```python
from build123d import *

# Parameters (mm, degrees)
FILLET1_R          = 0.75
CUT_EXTRUDE6_DEPTH = 3


with BuildPart() as part:
    # Sketch1 → Revolve1 (revolve)
    with BuildSketch(Plane(origin=(0, 0, 0), x_dir=(0, 0, -1), z_dir=(1, 0, 0))):
        with BuildLine():
            Line((0, 0), (140, 0))
            Line((140, 0), (140, 4.75))
            Line((140, 4.75), (6.25, 4.75))
            Line((6.25, 4.75), (6.25, 8.15))
            ThreePointArc((6.25, 8.15), (1.742375921, 5.135294539), (0, 0))
        make_face()
    revolve(axis=Axis((0, 0, 0), (0, 0, -1)))

    # Fillet1
    fillet1_edges = [part.edges().sort_by_distance(p)[0] for p in [
        (0, -8.15, -6.25),
        (0, -4.75, -140),
    ]]
    fillet(fillet1_edges, radius=FILLET1_R)

    # Sketch4 → Cut-Extrude6 (cut)
    with BuildSketch(Plane.XY):
        with BuildLine():
            Line((1.875, -3.247595264), (1.875, -9.329244328))
            Line((1.875, -9.329244328), (-1.875, -9.329244328))
            Line((-1.875, -9.329244328), (-1.875, -3.247595264))
            ThreePointArc((-1.875, -3.247595264), (-3.75, 0), (-1.875, 3.247595264))
            Line((-1.875, 3.247595264), (-1.875, 9.329244328))
            Line((-1.875, 9.329244328), (1.875, 9.329244328))
            Line((1.875, 9.329244328), (1.875, 3.247595264))
            ThreePointArc((1.875, 3.247595264), (3.75, 0), (1.875, -3.247595264))
        make_face()
    extrude(amount=-CUT_EXTRUDE6_DEPTH, mode=Mode.SUBTRACT)


solid = part.part
```
Can you work these out from the model? Positions are in its coordinate system, mm. A direction names the side the tool comes from. Round coordinates to 2 decimals unless told otherwise and drop trailing zeros. Loops run counter-clockwise (first coordinate to the right, second up) from the corner with the lowest first, then second, coordinate; pieces in that order, holes last. Notation, with made-up numbers: (65.25, 40.5) -> (87.25, 40.5) arc R21 ccw to (87.25, 68.5) -> close; hole circle Ø7 at (-21.5, -22). An arc over 180 degrees is marked (long way). One line per item, written item: value. Start each with the question number.
1. For faces 1 (the cylindrical face through (3.75, 0.05, -1.92)), 2 (the flat face through (-5, 1, -6.25)), 3 (the flat face through (-1.875, 4, -2)), which set-ups out of +Z, -Z, +X, -X, +Y, -Y let a thin tool reach every point of the face, with its end or its side?
2. If we section it at A-A, the plane z = -98: Write out the boundary of the cut face in (x, y).
3. For pin 1 (6 mm diameter, centred on y = -3.5, z = -96, fed in from +X); pin 2 (1.5 mm diameter, centred on x = 0, z = -85.5, fed in from -Y); pin 3 (2.5 mm diameter, centred on y = 5.5, z = -2.5, fed in from -X), each with a flat end and sliding along its axis, tell me the tip position at first contact or that it passes through.
4. If I drill on probe 1 along Y at (x, z) = (0.25, -9.5); probe 2 along Z at (x, y) = (3.25, -1.25); probe 3 along X at (y, z) = (-0.5, -103), over which ranges is the centre line in solid material (lowest first)?
5. If we mould it in two halves opening along X, with no side actions, what happens to faces 4 (the flat face through (0, 0, -140)), 5 (the cylindrical face through (-4.214, 2.192, -71.819)), 6 (the cylindrical face through (-3.75, -0.05, -1.92))? For each: pulls with the +X half, pulls with the -X half, needs draft (parallel to the pull), parting line crosses it, or undercut.
Calculated:
1. face 1: +Z
1. face 2: -Z
1. face 3: +Z, +Y, -Y
2. outline: circle Ø9.5 at (0, 0)
3. pin 1: stops at x = 4.72
3. pin 2: stops at y = -4.75
3. pin 3: stops at x = -4.94
4. probe 1: y = -4.74 to 4.74
4. probe 2: z = -140 to -3
4. probe 3: x = -4.72 to 4.72
5. face 4: needs draft
5. face 5: parting line crosses it
5. face 6: undercut
